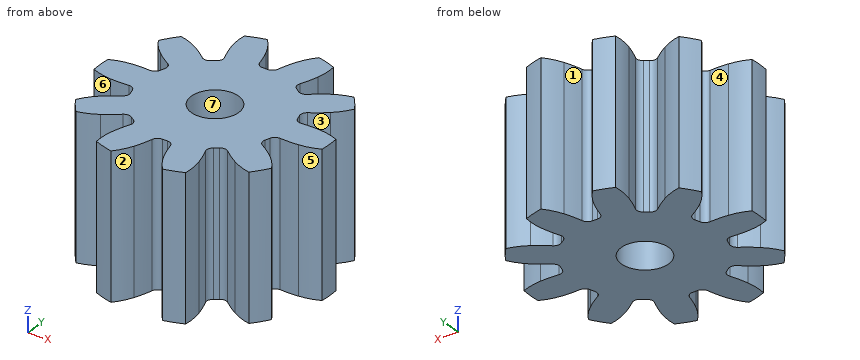
```python
from build123d import *

# Parameters (mm, degrees)
SKETCH1_R           = 7.62
ROUND_STOCK_DEPTH   = 4.7625
SINGLE_TOOTH_DEPTH  = 10.525
TOOTH_PATTERN_COUNT = 10
SKETCH5_R           = 1.5748
CUT_EXTRUDE1_DEPTH  = 10.525


with BuildPart() as part:
    # Sketch1 → Round Stock (new body, symmetric)
    with BuildSketch(Plane.XY):
        Circle(SKETCH1_R)
    extrude(amount=ROUND_STOCK_DEPTH, both=True)

    # Sketch2 → Single Tooth (cut, through all)
    with BuildSketch(Plane.XY.offset(4.7625)):
        with BuildLine():
            ThreePointArc((-6.527946851, -3.930688223), (-7.247050654, -2.354709497), (-7.59162051, -0.657037315))
            ThreePointArc((-7.59162051, -0.657037315), (-6.946040634, -0.884136963), (-6.271150147, -0.997585))
            ThreePointArc((-6.271150147, -0.997585), (-5.655082128, -1.02259203), (-5.038991647, -0.998144603))
            ThreePointArc((-5.038991647, -0.998144603), (-4.750649746, -1.075701008), (-4.576435033, -1.318199012))
            ThreePointArc((-4.576435033, -1.318199012), (-4.529406659, -1.471693436), (-4.477231654, -1.623515618))
            ThreePointArc((-4.477231654, -1.623515618), (-4.475637567, -1.922101463), (-4.663324555, -2.15432903))
            ThreePointArc((-4.663324555, -2.15432903), (-5.17612206, -2.496679544), (-5.659832794, -2.879026353))
            ThreePointArc((-5.659832794, -2.879026353), (-6.139147584, -3.367498418), (-6.527946851, -3.930688223))
        make_face()
    single_tooth = extrude(amount=-SINGLE_TOOTH_DEPTH, mode=Mode.SUBTRACT)

    # Tooth Pattern: Single Tooth ×10 about axis
    tooth_pattern_axis = Axis((0, 0, 0), (0, 0, 1))
    for i in range(1, TOOTH_PATTERN_COUNT):
        add(single_tooth.rotate(tooth_pattern_axis, i * 360 / TOOTH_PATTERN_COUNT), mode=Mode.SUBTRACT)

    # Sketch5 → Cut-Extrude1 (cut, through all)
    with BuildSketch(Plane.XY.offset(4.7625)):
        Circle(SKETCH5_R)
    extrude(amount=-CUT_EXTRUDE1_DEPTH, mode=Mode.SUBTRACT)


solid = part.part
```
Can you work these out from the model? Positions are in its coordinate system, mm. Face numbers are marked on the shaded views. A direction names the side the tool comes from. Round coordinates to 2 decimals unless told otherwise and drop trailing zeros. Loops run counter-clockwise (first coordinate to the right, second up) from the corner with the lowest first, then second, coordinate; pieces in that order, holes last.
Item 1: Suppose I cut it at B-B, the plane x = -6. Write out the boundary of the cut face in (y, z), then the cut area to 3 significant figures.
Item 2: If we mould it in two halves opening along X, with no side actions, what happens to the marked faces 4, 5, 6 and 7? For each: +X half, -X half, draft (parallel to the pull), parting line (faces both ways), or undercut.
Item 3: Suppose I cut it at C-C, the plane y = 2.5. Write out the boundary of the cut face in (x, z), then the cut area to 3 significant figures.
Item 4: Suppose I cut it at A-A, the plane y = 0. Write out the boundary of the cut face in (x, z).
Item 5: Will these pins go through, and if not, where does the flat tip stop? pin 1 Ø4 at (x, z) = (4.5, 0) entering from +Y; pin 2 Ø1 at (y, z) = (3.5, -2) entering from +X; pin 3 Ø2 at (x, z) = (-1.5, -0.5) entering from +Y.
Item 6: Please list where these lines run through material, in increasing order: L1, parallel to Y at x = 0, z = 4; L2, parallel to X at y = 4, z = 2; L3, parallel to X at y = 3.75, z = 2.
Item 7: Which directions (+Z, -Z, +X, -X, +Y, -Y) give clear straight access to the entire face, cutting with the end or side of a thin tool? Please do the marked faces 1, 2 and 3.
Reported:
1. outline: (-4.7, -4.76) - (-3.21, -4.76) - (-3.21, 4.76) - (-4.7, 4.76) - close; (-1.01, -4.76) - (1.01, -4.76) - (1.01, 4.76) - (-1.01, 4.76) - close; (3.21, -4.76) - (4.7, -4.76) - (4.7, 4.76) - (3.21, 4.76) - close
1. area: 47.7 mm2
2. face 4: undercut
2. face 5: +X half
2. face 6: -X half
2. face 7: undercut
3. outline: (-5.18, -4.76) - (5.18, -4.76) - (5.18, 4.76) - (-5.18, 4.76) - close
3. area: 98.7 mm2
4. outline: (-7.62, -4.76) - (-1.57, -4.76) - (-1.57, 4.76) - (-7.62, 4.76) - close; (1.57, -4.76) - (7.62, -4.76) - (7.62, 4.76) - (1.57, 4.76) - close
5. pin 1: stops at y = 7.2
5. pin 2: stops at x = 6.53
5. pin 3: stops at y = 7.42
6. L1: y = -4.76 to -1.57, 1.57 to 4.76
6. L2: x = -6.49 to -3.77, -2.6 to 2.6, 3.77 to 6.49
6. L3: x = -6.42 to -3.47, -2.94 to 2.94, 3.47 to 6.42
7. face 1: +Z, -Z, +Y
7. face 2: +Z, -Z, -Y
7. face 3: +Z, -Z, +X
